from build123d import *

# Parameters (mm, degrees)
SKETCH_2_R               = 90
EXTRUDE_1_DEPTH          = 4
CUT_EXTRUDE_1_DEPTH      = 128.342059038
CUT_EXTRUDE_1_DEPTH_BACK = 10
CUT_EXTRUDE_2_DEPTH      = 1
CUT_EXTRUDE_2_DEPTH_BACK = 1
SKETCH_2_8_R             = 30
CUT_EXTRUDE_4_DEPTH      = 124.190655084
CUT_EXTRUDE_5_DEPTH      = 1
CUT_EXTRUDE_5_DEPTH_BACK = 1
SKETCH_2_9_W             = 75.7
SKETCH_2_9_H             = 60.7
CUT_EXTRUDE_6_DEPTH      = 1
CUT_EXTRUDE_6_DEPTH_BACK = 1
SKETCH_2_10_R            = 17.5


with BuildPart() as part:
    # Sketch 2 → Extrude 1 (new body)
    with BuildSketch(Plane(origin=(0, 0, 0), x_dir=(1, 0, 0), z_dir=(0, 1, 0))):
        with Locations(Location((0, 0, 0), (0, 0, 270))):
            Circle(SKETCH_2_R)
    extrude(amount=EXTRUDE_1_DEPTH)

    # Sketch 2_5 → Cut-Extrude 1 (cut, two sides: drawn at the far end of the back side and taken through both)
    with BuildSketch(Plane(origin=(0, 0, 0), x_dir=(1, 0, 0), z_dir=(0, 1, 0)).offset(-CUT_EXTRUDE_1_DEPTH_BACK)):
        with BuildLine():
            Line((-69.717716958, 32.25), (-84.023434231, 32.25))
            ThreePointArc((-84.023434231, 32.25), (-90, 0), (-84.023434231, -32.25))
            Line((-84.023434231, -32.25), (-69.717716958, -32.25))
            Line((-69.717716958, -32.25), (-69.717716958, -11.341017113))
            Line((-69.717716958, -11.341017113), (-69.717716958, 32.25))
        make_face()
        with BuildLine():
            Line((84.023434231, 32.25), (69.717716958, 32.25))
            Line((69.717716958, 32.25), (69.717716958, -11.341017113))
            Line((69.717716958, -11.341017113), (69.717716958, -32.25))
            Line((69.717716958, -32.25), (84.023434231, -32.25))
            ThreePointArc((84.023434231, -32.25), (88.493245733, -16.399556689), (90, 0))
            ThreePointArc((90, 0), (88.493245733, 16.399556689), (84.023434231, 32.25))
        make_face()
    extrude(amount=CUT_EXTRUDE_1_DEPTH + CUT_EXTRUDE_1_DEPTH_BACK, mode=Mode.SUBTRACT)

    # Sketch 2_7 → Cut-Extrude 2 (cut, two sides: drawn at the far end of the back side and taken through both)
    with BuildSketch(Plane(origin=(0, 0, 0), x_dir=(1, 0, 0), z_dir=(0, 1, 0)).offset(-CUT_EXTRUDE_2_DEPTH_BACK)):
        Polygon((-69.717716958, 54.158982887), (-69.717716958, 32.25), (-69.717716958, -11.341017113), (-47.317716958, -11.341017113), (-47.317716958, 54.158982887), align=None)
        Polygon((69.717716958, -11.341017113), (69.717716958, 32.25), (69.717716958, 54.158982887), (47.317716958, 54.158982887), (47.317716958, -11.341017113), align=None)
    extrude(amount=CUT_EXTRUDE_2_DEPTH + CUT_EXTRUDE_2_DEPTH_BACK, mode=Mode.SUBTRACT)

    # Sketch 2_8 → Cut-Extrude 4 (cut, through all)
    with BuildSketch(Plane(origin=(0, 0, 0), x_dir=(1, 0, 0), z_dir=(0, 1, 0))):
        with Locations(Location((0, 18.868843399, 0), (0, 0, 270))):
            Circle(SKETCH_2_8_R)
    extrude(amount=CUT_EXTRUDE_4_DEPTH, mode=Mode.SUBTRACT)

    # Sketch 2_9 → Cut-Extrude 5 (cut, two sides: drawn at the far end of the back side and taken through both)
    with BuildSketch(Plane(origin=(0, 0, 0), x_dir=(1, 0, 0), z_dir=(0, 1, 0)).offset(-CUT_EXTRUDE_5_DEPTH_BACK)):
        with Locations((0, -46.344841494)):
            Rectangle(SKETCH_2_9_W, SKETCH_2_9_H)
    extrude(amount=CUT_EXTRUDE_5_DEPTH + CUT_EXTRUDE_5_DEPTH_BACK, mode=Mode.SUBTRACT)

    # Sketch 2_10 → Cut-Extrude 6 (cut, two sides: drawn at the far end of the back side and taken through both)
    with BuildSketch(Plane(origin=(0, 0, 0), x_dir=(1, 0, 0), z_dir=(0, 1, 0)).offset(-CUT_EXTRUDE_6_DEPTH_BACK)):
        with Locations(Location((0, 71.575794202, 0), (0, 0, 270))):
            Circle(SKETCH_2_10_R)
    extrude(amount=CUT_EXTRUDE_6_DEPTH + CUT_EXTRUDE_6_DEPTH_BACK, mode=Mode.SUBTRACT)


solid = part.part
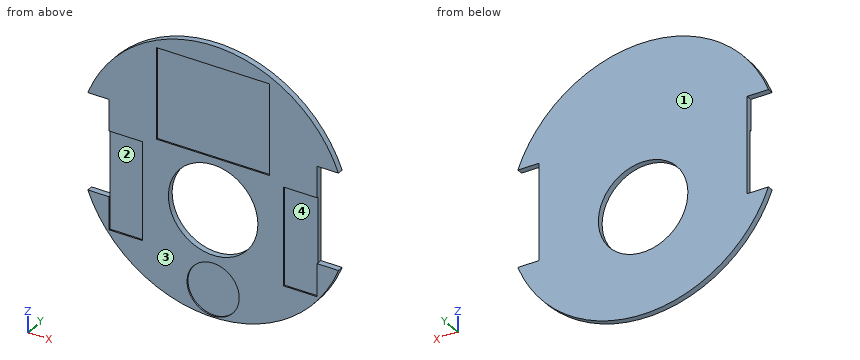
Geometry: final body of the model. Coordinates: model frame, mm. Face numbers are marked on the shaded views. A direction names the side the tool comes from. Round coordinates to 2 decimals unless told otherwise and drop trailing zeros. Loops run counter-clockwise (first coordinate to the right, second up) from the corner with the lowest first, then second, coordinate; pieces in that order, holes last.
Q1. Section C-C on z = -46.5. Return loops of the section in (x, y), plus the area to 3 significant figures.
Q2. Pin query (flat end, axial travel): P1, Ø0.8, axis at x = 62.5, y = 0.5, coming from the -Z side; P2, Ø17.5, axis at x = 0, z = -76.5, coming from the -Y side; P3, Ø1.1, axis at y = 0.5, z = -40, coming from the -X side. Return the tip coordinate at first contact, or that it passes through.
Q3. Section B-B on y = 2.95. Return loops of the section in (x, z).
Q4. Section A-A on x = 0. Return loops of the section in (y, z), plus the area to 3 significant figures.
Q5. Access query for the marked faces 3 and 4. Directions: +Z, -Z, +X, -X, +Y, -Y. A direction counts if a zero-diameter tool reaches every point of the face in a straight line with its end or side. Return the directions, or none.
Q6. Section D-D on z = 29.5. Return loops of the section in (x, y).
Q7. Pull-direction query (X, two-part tool) for the marked faces 1 and 2; classes: released by +X, released by -X, zero draft, split by the parting line, or undercut.
Q8. Material intervals for L1, parallel to Z at x = 0, y = 0.45; L2, parallel to Y at x = -18.5, z = 65.5; L3, parallel to X at y = 3, z = 24, sorted ascending.
Evaluation:
1. outline: (-77.06, 0) - (-69.72, 0) - (-69.72, 1) - (-47.32, 1) - (-47.32, 0) - (-11.68, 0) - (-11.68, 4) - (-77.06, 4) - close; (11.68, 0) - (47.32, 0) - (47.32, 1) - (69.72, 1) - (69.72, 0) - (77.06, 0) - (77.06, 4) - (11.68, 4) - close
1. area: 478 mm2
2. P1: stops at z = -65.14
2. P2: stops at y = 1
2. P3: stops at x = -80.89
3. outline: (-84.02, -32.25) arc R90 ccw to (84.02, -32.25) - (69.72, -32.25) - (69.72, 32.25) - (84.02, 32.25) arc R90 ccw to (-84.02, 32.25) - (-69.72, 32.25) - (-69.72, -32.25) - close; hole circle Ø60 at (0, -18.87)
4. outline: (0, -90) - (4, -90) - (4, -48.87) - (0, -48.87) - (0, -54.08) - (1, -54.08) - (1, -89.08) - (0, -89.08) - close; (0, 11.13) - (4, 11.13) - (4, 90) - (0, 90) - (0, 76.69) - (1, 76.69) - (1, 15.99) - (0, 15.99) - close
4. area: 384 mm2
5. face 3: +Z, -Z, +X, -X, -Y
5. face 4: -Y
6. outline: (-69.72, 0) - (-37.85, 0) - (-37.85, 1) - (37.85, 1) - (37.85, 0) - (69.72, 0) - (69.72, 4) - (-69.72, 4) - close
7. face 1: zero draft
7. face 2: undercut
8. L1: z = -90 to -89.08, -54.08 to -48.87, 11.13 to 15.99, 76.69 to 90
8. L2: y = 1 to 4
8. L3: x = -69.72 to 69.72
